from build123d import *

# Parameters (mm, degrees)
BOSS_EXTRUDE1_DEPTH = 117
SKETCH2_W           = 117
SKETCH2_H           = 5.816025404
BOSS_EXTRUDE2_DEPTH = 1.5
SKETCH3_W           = 117
SKETCH3_H           = 4.95
BOSS_EXTRUDE3_DEPTH = 1.5
SKETCH4_W           = 7
SKETCH4_H           = 0.5
CUT_EXTRUDE1_DEPTH  = 120.168326329
DRAFT1_ANGLE        = 30
DRAFT2_ANGLE        = 30
DRAFT3_ANGLE        = 45
HOLE1_D             = 6
HOLE1_DEPTH         = 20.3
HOLE1_CBORE_D       = 9.5
HOLE1_CBORE_DEPTH   = 8.5
CHAMFER1_SIZE       = 1
CHAMFER2_SIZE       = 0.404011753
CHAMFER2_SIZE_2     = 0.538175706
FILLET1_R           = 0.5


with BuildPart() as part:
    # Sketch1 → Boss-Extrude1 (new body)
    with BuildSketch(Plane(origin=(58.5, 0, 0), x_dir=(0, 0, -1), z_dir=(1, 0, 0))):
        with BuildLine():
            Line((-8.5, 0), (8.5, 0))
            Line((8.5, 0), (8.5, 9.005088936))
            ThreePointArc((8.5, 9.005088936), (7.111244718, 9.113338811), (6.503340774, 10.366659226))
            Line((6.503340774, 10.366659226), (6, 10.87))
            Line((6, 10.87), (6, 14.93))
            Line((6, 14.93), (6.503340774, 15.433340774))
            ThreePointArc((6.503340774, 15.433340774), (7.111244718, 16.686661189), (8.5, 16.794911064))
            Line((8.5, 16.794911064), (8.5, 20.3))
            Line((8.5, 20.3), (-8.5, 20.3))
            Line((-8.5, 20.3), (-8.5, 16.794911064))
            ThreePointArc((-8.5, 16.794911064), (-7.111244718, 16.686661189), (-6.503340774, 15.433340774))
            Line((-6.503340774, 15.433340774), (-6, 14.93))
            Line((-6, 14.93), (-6, 10.87))
            Line((-6, 10.87), (-6.503340774, 10.366659226))
            ThreePointArc((-6.503340774, 10.366659226), (-7.111244718, 9.113338811), (-8.5, 9.005088936))
            Line((-8.5, 9.005088936), (-8.5, 0))
        make_face()
    extrude(amount=-BOSS_EXTRUDE1_DEPTH)

    # Sketch2 → Boss-Extrude2 (add)
    with BuildSketch(Plane(origin=(0, 0, -8.5), x_dir=(-1, 0, 0), z_dir=(0, 0, -1))):
        with Locations((0, 2.908012702)):
            Rectangle(SKETCH2_W, SKETCH2_H)
    extrude(amount=BOSS_EXTRUDE2_DEPTH)

    # Sketch3 → Boss-Extrude3 (add)
    with BuildSketch(Plane.XY.offset(8.5)):
        with Locations((0, 2.475)):
            Rectangle(SKETCH3_W, SKETCH3_H)
    extrude(amount=BOSS_EXTRUDE3_DEPTH)

    # Sketch4 → Cut-Extrude1 (cut, through all)
    with BuildSketch(Plane.ZY.offset(58.5)):
        with Locations((0, 0.25)):
            Rectangle(SKETCH4_W, SKETCH4_H)
    extrude(amount=-CUT_EXTRUDE1_DEPTH, mode=Mode.SUBTRACT)

    # Draft1
    draft1_faces = [part.faces().sort_by_distance(p)[0] for p in [
        (0, 4.95, 9.25),
    ]]
    draft(draft1_faces, Plane.XY.offset(10), DRAFT1_ANGLE)

    # Draft2
    draft2_faces = [part.faces().sort_by_distance(p)[0] for p in [
        (0, 5.816025404, -9.25),
    ]]
    draft(draft2_faces, Plane(origin=(-58.5, 0, -8.5), x_dir=(0, -1, 0), z_dir=(0, 0, -1)), DRAFT2_ANGLE)

    # Draft3
    draft3_faces = [part.faces().sort_by_distance(p)[0] for p in [
        (0, 0.25, 3.5),
        (0, 0.25, -3.5),
    ]]
    draft(draft3_faces, Plane(origin=(58.5, 0.5, 3.5), x_dir=(0, 0, -1), z_dir=(0, -1, 0)), DRAFT3_ANGLE)

    # Hole1
    with Locations(Plane(origin=(0, 20.3, 0), x_dir=(-1, 0, 0), z_dir=(0, 1, 0))):
        with Locations((38.5, 0), (-21.5, 0)):
            CounterBoreHole(HOLE1_D / 2, HOLE1_CBORE_D / 2, HOLE1_CBORE_DEPTH, depth=HOLE1_DEPTH)

    # Chamfer1
    chamfer1_edges = [part.edges().sort_by_distance(p)[0] for p in [
        (0, 20.3, 8.5),
        (0, 20.3, -8.5),
        (0, 0, -10),
        (0, 0, 10),
    ]]
    chamfer(chamfer1_edges, length=CHAMFER1_SIZE)

    # Chamfer2
    # the kernel refuses this chamfer: 0.538175706, 0.404011753 mm, written as the material it takes off along each edge
    with BuildSketch(Plane(origin=(60.548293872, 9.005088936, 8.5), x_dir=(0, -0.15244489299056474, -0.9883119723048464), z_dir=(-1, 0, 0))) as chamfer2_piece_1:
        with BuildLine():
            Line((0.800315903, 0), (CHAMFER2_SIZE * 0.152444893097, CHAMFER2_SIZE * 0.988311972993))
            Line((CHAMFER2_SIZE * 0.152444893097, CHAMFER2_SIZE * 0.988311972993), (0, 0))
            ThreePointArc((0, 0), (0.41007662, 0.05837118), (0.800315903, 0))
        make_face()
    extrude(amount=121.096587744, mode=Mode.SUBTRACT)
    with BuildSketch(Plane(origin=(59.884017308, 16.794911064, 8.5), x_dir=(0, 1, 0), z_dir=(-1, 0, 0))) as chamfer2_piece_2:
        with BuildLine():
            Line((CHAMFER2_SIZE_2, 0), (0.122854653, 0.415321053))
            ThreePointArc((0.122854653, 0.415321053), (0.079061625, 0.207906373), (0, 0))
            Line((0, 0), (CHAMFER2_SIZE_2, 0))
        make_face()
    extrude(amount=119.768034616, mode=Mode.SUBTRACT)
    with BuildSketch(Plane(origin=(60.548293872, 16.794911064, -8.5), x_dir=(0, 1, 0), z_dir=(-1, 0, 0))) as chamfer2_piece_3:
        with BuildLine():
            Line((CHAMFER2_SIZE, 0), (0.122004072, -0.790961789))
            ThreePointArc((0.122004072, -0.790961789), (0.120203022, -0.396385245), (0, 0))
            Line((0, 0), (CHAMFER2_SIZE, 0))
        make_face()
    extrude(amount=121.096587744, mode=Mode.SUBTRACT)
    with BuildSketch(Plane(origin=(59.884017308, 9.005088936, -8.5), x_dir=(0, -0.28365649946208477, 0.958925956637381), z_dir=(-1, 0, 0))) as chamfer2_piece_4:
        with BuildLine():
            Line((0.433110659, 0), (CHAMFER2_SIZE_2 * 0.283656499578, -CHAMFER2_SIZE_2 * 0.958925957029))
            Line((CHAMFER2_SIZE_2 * 0.283656499578, -CHAMFER2_SIZE_2 * 0.958925957029), (0, 0))
            ThreePointArc((0, 0), (0.221793162, -0.01684025), (0.433110659, 0))
        make_face()
    extrude(amount=119.768034616, mode=Mode.SUBTRACT)

    # Fillet1
    fillet1_edges = [part.edges().sort_by_distance(p)[0] for p in [
        (0, 5.816025404, -8.5),
        (0, 5.816025404, 8.5),
    ]]
    fillet(fillet1_edges, radius=FILLET1_R)


solid = part.part
Design review of the part built by this model. Coordinates are the model's own, in mm. A direction names the side the tool comes from. Round coordinates to 2 decimals unless told otherwise and drop trailing zeros. Write each loop counter-clockwise with the first axis right and the second up, starting at its lowest first coordinate (ties: lowest second). Pieces come first, ordered by that corner, then holes. Notation, with made-up numbers: (64, 35.25) - (72, 35.25) arc R18 cw to (72, 52.25) - close; hole circle Ø7 at (86.25, 36.5). An arc over 180 degrees is marked (long way). Use a Markdown table: item, result. Add a question column.
1. Clearance check with flat-ended pins moving along their axes: pin 1 (8 mm diameter, centred on x = 21.5, z = 0, fed in from +Y); pin 2 (5.5 mm diameter, centred on x = -38.5, z = 0, fed in from +Y); pin 3 (1.7 mm diameter, centred on x = 11, y = 18, fed in from -Z); pin 4 (3 mm diameter, centred on x = 26.5, y = 8, fed in from +Z). State where each tip first meets the part, or that it passes through.
2. Wall thickness on probe 1 along Z at (x, y) = (21.5, 3.5); probe 2 along X at (y, z) = (7, 2.5); probe 3 along X at (y, z) = (15, -0.5): over which ranges is each line inside the solid? List them lowest first.
3. Mouldability with a two-part tool opening along Y and no side actions: class faces 1 (the face through (17.112, 16.11, -1.819)), 2 (the face through (-1, 0, -7)), 3 (the face through (1, 13, -6)), 4 (the face through (1, 13, 6)) as +Y half, -Y half, draft (parallel to the pull), parting line (faces both ways), or undercut.
4. We need section C-C (y = 3.25). State the section outline as (x, z) points.
5. We need section A-A (z = 0). State the section outline as (x, y) points, then the cut area to 3 significant figures.
6. For faces 5 (the face through (-42, 11.8, 0)), 6 (the face through (1, 18, -8.5)), 7 (the face through (1, 18, 8.5)), list the 3-axis set-ups (+Z, -Z, +X, -X, +Y, -Y) from which the entire face can be reached by the end or side of a thin tool; tool diameter is ignored.
Output:
| question | item | result |
|---|---|---|
| 1 | pin 1 | stops at y = 11.8 |
| 1 | pin 2 | passes through |
| 1 | pin 3 | stops at z = -8.5 |
| 1 | pin 4 | stops at z = 8.5 |
| 2 | probe 1 | z = -10 to -3, 3 to 10 |
| 2 | probe 2 | x = -58.5 to -40.16, -36.84 to 19.84, 23.16 to 58.5 |
| 2 | probe 3 | x = -58.5 to -43.22, -33.78 to 16.78, 26.22 to 58.5 |
| 3 | face 1 | draft |
| 3 | face 2 | -Y half |
| 3 | face 3 | undercut |
| 3 | face 4 | undercut |
| 4 | outline | (-58.5, -10) - (58.5, -10) - (58.5, 10) - (-58.5, 10) - close; hole circle Ø6 at (-38.5, 0); hole circle Ø6 at (21.5, 0) |
| 5 | outline | (-58.5, 0.5) - (-41.5, 0.5) - (-41.5, 11.8) - (-43.25, 11.8) - (-43.25, 20.3) - (-58.5, 20.3) - close; (-35.5, 0.5) - (18.5, 0.5) - (18.5, 11.8) - (16.75, 11.8) - (16.75, 20.3) - (-33.75, 20.3) - (-33.75, 11.8) - (-35.5, 11.8) - close; (24.5, 0.5) - (58.5, 0.5) - (58.5, 20.3) - (26.25, 20.3) - (26.25, 11.8) - (24.5, 11.8) - close |
| 5 | area | 2,020 mm2 |
| 6 | face 5 | +Y |
| 6 | face 6 | -Z, +X, -X, +Y |
| 6 | face 7 | +Z, +X, -X, +Y |
